```python
from build123d import *

# Parameters (mm, degrees)
BOSS_EXTRUDE1_DEPTH = 2.54
SKETCH4_W           = 0.135
SKETCH4_H           = 0.17696191
SKETCH4_W_2         = 6.45
SKETCH4_H_2         = 5.360645495


with BuildPart() as part:
    # Sketch2 → Boss-Extrude1 (new, symmetric)
    with BuildSketch(Plane.XY):
        Polygon((0, 3.166258563), (-8.153042882, 3.166258563), (-8.153042882, -5.723741437), (0, -5.723741437), (0, -0.430777301), (-0.971812772, -0.430777301), (-0.971812772, 2.100957578), (0, 2.100957578), align=None)
    extrude(amount=BOSS_EXTRUDE1_DEPTH, both=True)

    # Sketch4 → Cut-Revolve2 (revolve, cut)
    with BuildSketch(Plane.XY):
        with Locations((-0.0675, 2.60664071)):
            Rectangle(SKETCH4_W, SKETCH4_H)
        with Locations((-3.225, -3.111100048)):
            Rectangle(SKETCH4_W_2, SKETCH4_H_2)
    revolve(axis=Axis((0, 5.644041385, 0), (0, -1, 0)), mode=Mode.SUBTRACT)


solid = part.part
```
Check sheet for the modelled part. Datum: model origin and axes. Units: mm. A direction names the side the tool comes from. Give positions to 0.01 mm unless a question says otherwise; leave off trailing zeros. Write each loop counter-clockwise with the first axis right and the second up, starting at its lowest first coordinate (ties: lowest second). Pieces come first, ordered by that corner, then holes. Notation, with made-up numbers: (-11, -32.5) - (42, -32.5) arc R9 ccw to (42, -16.5) - close; hole circle Ø9 at (-15, 71). An arc over 180 degrees is marked (long way). Answer as a JSON object with one key per item and string values. Group by question number.
1) Sectioned sample at D-D (z = 0.65). Record the cut outline in (x, y), then the cut area to 3 significant figures.
2) Sectioned sample at A-A (z = 0). Record the cut outline in (x, y) (3 decimals), then the cut area to 3 significant figures.
3) Sectioned sample at B-B (y = 1.25). Record the cut outline in (x, z), then the cut area to 3 significant figures.
4) Release check for a two-part mould opening along Z. For faces 3 (the face through (-5, 0, 2.54)), 4 (the face through (-5, 0, -2.54)), 5 (the face through (-0.5, 2.101, 0)), 6 (the face through (-6.45, -3.04, 0.04)) record: pulls with the +Z half, pulls with the -Z half, needs draft (parallel to the pull), parting line crosses it, or undercut.
5) Access from +Z, -Z, +X, -X, +Y, -Y to the whole of each face (thin tool, end or side, straight path). Record for faces 1 (the face through (-0.972, 1, 0)), 2 (the face through (-8.153, -1, 0)).
6) Thickness scan on probe 1 along X at (y, z) = (0.75, -1.2); probe 2 along Y at (x, z) = (-4, -1.6); probe 3 along X at (y, z) = (-1, -0.1). Record the ranges inside material, lowest first. Write a range as from..to.
7) Depth check by flat-ended pin: P1, Ø3, axis at y = 0.5, z = -0.5, coming from the +X side; P2, Ø0.5, axis at x = 0, z = 0, coming from the -Y side; P3, Ø1.5, axis at x = -3.5, y = -1.5, coming from the -Z side; P4, Ø2.5, axis at x = -5, z = -0.5, coming from the -Y side. Enter the tip coordinate at first touch or a pass-through.
8) Sectioned sample at C-C (x = -0.75). Record the cut outline in (y, z), then the cut area to 3 significant figures.
Geometry results:
{
 "1": {"outline": "(-8.15, -5.72) - (-6.42, -5.72) - (-6.42, -0.43) - (-0.97, -0.43) - (-0.97, 2.1) - (0, 2.1) - (0, 3.17) - (-8.15, 3.17) - close", "area": "36.1 mm^2"},
 "2": {"outline": "(-8.153, -5.724) - (-6.45, -5.724) - (-6.45, -0.431) - (-0.972, -0.431) - (-0.972, 2.101) - (0, 2.101) - (0, 2.518) - (-0.135, 2.518) - (-0.135, 2.695) - (0, 2.695) - (0, 3.166) - (-8.153, 3.166) - close", "area": "35.9 mm^2"},
 "3": {"outline": "(-8.15, -2.54) - (-0.97, -2.54) - (-0.97, 2.54) - (-8.15, 2.54) - close", "area": "36.5 mm^2"},
 "4": {"face 3": "pulls with the +Z half", "face 4": "pulls with the -Z half", "face 5": "needs draft", "face 6": "undercut"},
 "5": {"face 1": "+Z, -Z, +X, -Y", "face 2": "+Z, -Z, -X, +Y, -Y"},
 "6": {"probe 1": "x = -8.15..-0.97", "probe 2": "y = -0.43..3.17", "probe 3": "x = -8.15..-6.45"},
 "7": {"P1": "stops at x = -0.97", "P2": "stops at y = 2.1", "P3": "passes through", "P4": "stops at y = -0.43"},
 "8": {"outline": "(2.1, -2.54) - (3.17, -2.54) - (3.17, 2.54) - (2.1, 2.54) - close", "area": "5.41 mm^2"}
}
